Part model, mm, in its own coordinate system. Face numbers are marked on the shaded views. Round coordinates to 2 decimals unless told otherwise and drop trailing zeros.
1) Flat gauge pins, fed straight in: pin 1 (5 mm diameter, centred on x = -63.5, y = 4.5, fed in from -Z); pin 2 (4 mm diameter, centred on x = -77.54, z = 44.77, fed in from +Y); pin 3 (2 mm diameter, centred on y = 10.5, z = 41.5, fed in from +X); pin 4 (1 mm diameter, centred on y = 12, z = -39, fed in from +X). Where does each tip first touch, or does it go through?
2) Drill centre lines: L1, parallel to Z at x = -77.5, y = -22; L2, parallel to Z at x = -80, y = -14; L3, parallel to Z at x = 63, y = 29. Where is each one in solid material? Low to high.
3) Saw through at A-A on y = -22.5. Count the separate pieces of the cut face and the enclosed holes in it, and give its area (3 significant figures).
4) Pull direction X, two halves, no side cores. Call the marked faces 1, 2 and 3: +X half, -X half, draft (parallel to the pull), parting line (faces both ways), or undercut.
```python
from build123d import *

# Parameters (mm, degrees)
SKETCH1_R           = 95.25
BOSS_EXTRUDE1_DEPTH = 34.925
SKETCH8_R           = 3.175
CUT_EXTRUDE1_DEPTH  = 69.85
CIRPATTERN1_COUNT   = 3
CUT_EXTRUDE2_START  = -34.925
SKETCH12_R          = 3.175
CUT_EXTRUDE2_DEPTH  = 63.5
CIRPATTERN2_COUNT   = 3


# Read off the part's stored shape, not the designer's step: Cavity1
with BuildPart() as part:
    # Sketch1 → Boss-Extrude1 (new, symmetric)
    with BuildSketch(Plane(origin=(0, 0, 0), x_dir=(1, 0, 0), z_dir=(0, 1, 0))):
        with Locations(Location((0, 0, 0), (0, 0, 270))):
            Circle(SKETCH1_R)
    extrude(amount=BOSS_EXTRUDE1_DEPTH, both=True)

    # Cavity1 outline → Cavity1 (revolve, cut)
    with BuildSketch(Plane.XY):
        with BuildLine():
            Line((0, 34.925), (0, -28.752211277))
            Line((0, -28.752211277), (0.381787731, -28.752211277))
            ThreePointArc((0.381787731, -28.752211277), (9.972417265, -27.913139917), (19.271640373, -25.421420595))
            Line((19.271640373, -25.421420595), (49.189756576, -14.532116831))
            ThreePointArc((49.189756576, -14.532116831), (74.301764107, 4.737004269), (83.820002599, 34.925))
            Line((83.820002599, 34.925), (0, 34.925))
        make_face()
    revolve(axis=Axis((0, 0, 0), (0, 1, 0)), mode=Mode.SUBTRACT)

    # Sketch8 → Cut-Extrude1 (cut)
    with BuildSketch(Plane(origin=(0, 34.925, 0), x_dir=(1, 0, 0), z_dir=(0, 1, 0))):
        with Locations(Location((0, 89.535, 0), (0, 0, 270))):
            Circle(SKETCH8_R)
    cut_extrude1 = extrude(amount=-CUT_EXTRUDE1_DEPTH, mode=Mode.SUBTRACT)

    # CirPattern1: Cut-Extrude1 ×3 about axis
    cirpattern1_axis = Axis((0, 0, 0), (0, 1, 0))
    for i in range(1, CIRPATTERN1_COUNT):
        add(cut_extrude1.rotate(cirpattern1_axis, i * 360 / CIRPATTERN1_COUNT), mode=Mode.SUBTRACT)

    # Sketch12 → Cut-Extrude2 (cut)
    with BuildSketch(Plane(origin=(0, 34.925, 0), x_dir=(1, 0, 0), z_dir=(0, 1, 0)).offset(CUT_EXTRUDE2_START)):
        with Locations(Location((77.539584528, 44.7675, 0), (0, 0, 270))):
            Circle(SKETCH12_R)
    cut_extrude2 = extrude(amount=-CUT_EXTRUDE2_DEPTH, mode=Mode.SUBTRACT)

    # CirPattern2: Cut-Extrude2 ×3 about axis
    cirpattern2_axis = Axis((0, 0, 0), (0, 1, 0))
    for i in range(1, CIRPATTERN2_COUNT):
        add(cut_extrude2.rotate(cirpattern2_axis, i * 360 / CIRPATTERN2_COUNT), mode=Mode.SUBTRACT)


solid = part.part
```
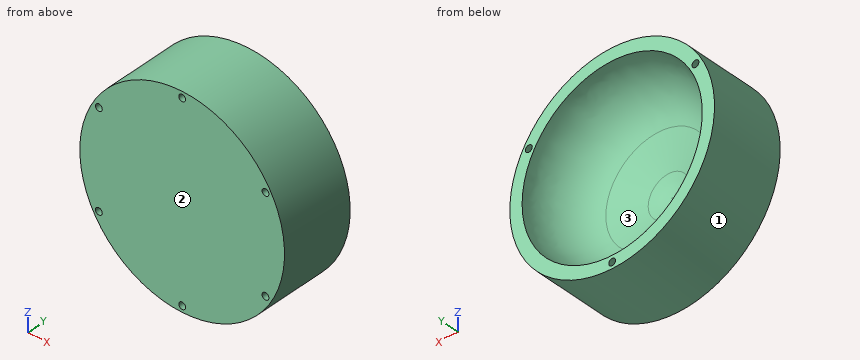
Completed:
1. pin 1: stops at z = -73.15
1. pin 2: passes through
1. pin 3: stops at x = 86.21
1. pin 4: stops at x = 87.12
2. L1: z = -55.37 to -47.94, -41.59 to 41.59, 47.94 to 55.37
2. L2: z = -51.7 to -46.77, -42.76 to 42.76, 46.77 to 51.7
2. L3: z = -71.44 to -54.78, 54.78 to 71.44
3. separate pieces: 1
3. enclosed holes: 7
3. area: 26,000 mm2
4. face 1: parting line
4. face 2: draft
4. face 3: undercut
